Here's how the part is built. I have some questions about the finished solid (model axes, mm). Round coordinates to 2 decimals unless told otherwise and drop trailing zeros. Write each loop counter-clockwise with the first axis right and the second up, starting at its lowest first coordinate (ties: lowest second). Pieces come first, ordered by that corner, then holes. Notation, with made-up numbers: (54.5, 11) -> (75.5, 11) arc R14 cw to (75.5, 23) -> close; hole circle Ø8 at (-25, -5.5). An arc over 180 degrees is marked (long way). Put each result on its own line as item: value. Start each with the question number.
1) If I drill on line 1 along X through (y, z) = (37.5, 9.9); line 2 along Y through (x, z) = (39.5, 12.7); line 3 along Y through (x, z) = (9.5, 11.75), over which ranges is the centre line in solid material (lowest first)? Write a range as [from, to].
2) I want a section at D-D, the plane x = 44. List the corners of the cut face in (y, z) for me, then the cut area to 3 significant figures.
3) I want a section at A-A, the plane x = 19. List the corners of the cut face in (y, z) for me.
4) I want a section at B-B, the plane z = 9.5. Give the number of separate pieces and of enclosed holes in the cut face, then the cut area to 3 significant figures.
5) Will these pins go through, and if not, where does the flat tip stop? P1, Ø0.6, axis at y = 3, z = 9, coming from the +X side; P2, Ø1, axis at y = 38, z = 9, coming from the -X side; P3, Ø3, axis at x = 34, y = 31, coming from the -Z side.
6) I want a section at C-C, the plane x = 106.5. List the corners of the cut face in (y, z) for me.
from build123d import *

# Parameters (mm, degrees)
SKETCH005_W     = 115
SKETCH005_H     = 40
PAD002_DEPTH    = 1
SKETCH006_W     = 5
SKETCH006_H     = 2
PAD003_DEPTH    = 5
SKETCH007_R     = 2
POCKET002_DEPTH = 5
SKETCH008_W     = 26
SKETCH008_H     = 18
POCKET003_DEPTH = 5
SKETCH009_W     = 15
SKETCH009_H     = 3.2
POCKET004_DEPTH = 5
SKETCH010_R     = 1.2
POCKET005_DEPTH = 38.701
FILLET002_R     = 2


with BuildPart() as part:
    # Sketch005 → Pad002 (new body)
    with BuildSketch(Plane.XY):
        with Locations((57.5, 20)):
            Rectangle(SKETCH005_W, SKETCH005_H)
    extrude(amount=PAD002_DEPTH)

    # Sketch006 → Pad003 (join)
    with BuildSketch(Plane(origin=(0, 0, 0), x_dir=(1, 0, 0), z_dir=(0, 0, -1))):
        with Locations((8.5, -2.3)):
            Rectangle(SKETCH006_W, SKETCH006_H)
        with Locations((106.5, -2.3)):
            Rectangle(SKETCH006_W, SKETCH006_H)
        with Locations((106.5, -37.7)):
            Rectangle(SKETCH006_W, SKETCH006_H)
        with Locations((8.5, -37.7)):
            Rectangle(SKETCH006_W, SKETCH006_H)
    extrude(amount=PAD003_DEPTH)

    # Sketch007 (on Face5 of Pad003) → Pocket002 (cut)
    with BuildSketch(Plane.XY.offset(1)):
        with Locations((60.085, 10.835)):
            Circle(SKETCH007_R)
        with Locations((60.085, 26.085)):
            Circle(SKETCH007_R)
        with Locations((74.085, 18.585)):
            Circle(SKETCH007_R)
        with Locations((88.085, 18.585)):
            Circle(SKETCH007_R)
    extrude(amount=-POCKET002_DEPTH, mode=Mode.SUBTRACT)

    # Sketch008 (on Face5 of Pocket002) → Pocket003 (cut)
    with BuildSketch(Plane.XY.offset(1)):
        with Locations((37.75, 19.9)):
            Rectangle(SKETCH008_W, SKETCH008_H)
    extrude(amount=-POCKET003_DEPTH, mode=Mode.SUBTRACT)

    # Sketch009 (on Face5 of Pocket003) → Pocket004 (cut)
    with BuildSketch(Plane.XY.offset(1)):
        with Locations((19.95, 35.87)):
            Rectangle(SKETCH009_W, SKETCH009_H)
    extrude(amount=-POCKET004_DEPTH, mode=Mode.SUBTRACT)

    # Sketch010 (on Face7 of Pocket004) → Pocket005 (cut, through all)
    with BuildSketch(Plane.XZ.offset(-1.3)):
        with Locations((8.5, -2.5)):
            Circle(SKETCH010_R)
        with Locations((106.5, -2.5)):
            Circle(SKETCH010_R)
    extrude(amount=-POCKET005_DEPTH, mode=Mode.SUBTRACT)

    # Fillet002
    fillet002_edges = [part.edges().sort_by_distance(p)[0] for p in [
        (0, 0, 0.5),
        (115, 0, 0.5),
        (115, 40, 0.5),
        (0, 40, 0.5),
    ]]
    fillet(fillet002_edges, radius=FILLET002_R)


with BuildPart() as part_1:
    # Body001 placement: moved
    add(part.part.moved(Location((0, 0, 12))))


solid = part_1.part
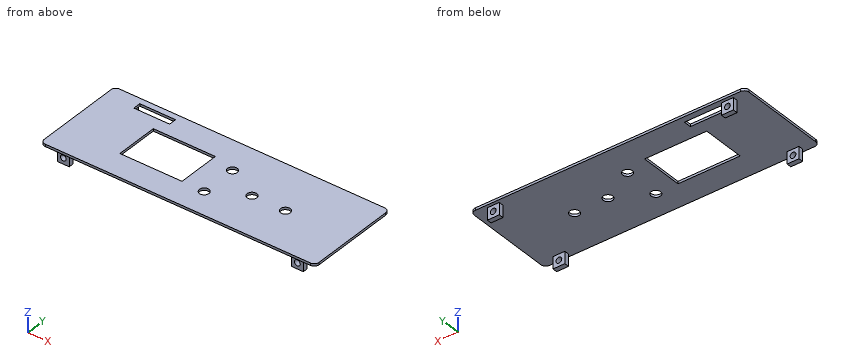
Findings:
1. line 1: x = [6, 7.37], [9.63, 11], [104, 105.37], [107.63, 109]
1. line 2: y = [0, 10.9], [28.9, 40]
1. line 3: y = [1.3, 3.3], [36.7, 38.7]
2. outline: (0, 12) -> (10.9, 12) -> (10.9, 13) -> (0, 13) -> close; (28.9, 12) -> (40, 12) -> (40, 13) -> (28.9, 13) -> close
2. area: 22.0 mm2
3. outline: (0, 12) -> (34.27, 12) -> (34.27, 13) -> (0, 13) -> close; (37.47, 12) -> (40, 12) -> (40, 13) -> (37.47, 13) -> close
4. separate pieces: 8
4. enclosed holes: 0
4. area: 20.8 mm2
5. P1: stops at x = 109
5. P2: stops at x = 6
5. P3: stops at z = 12
6. outline: (0, 12) -> (1.3, 12) -> (1.3, 10.7) -> (3.3, 10.7) -> (3.3, 12) -> (36.7, 12) -> (36.7, 10.7) -> (38.7, 10.7) -> (38.7, 12) -> (40, 12) -> (40, 13) -> (0, 13) -> close; (1.3, 7) -> (3.3, 7) -> (3.3, 8.3) -> (1.3, 8.3) -> close; (36.7, 7) -> (38.7, 7) -> (38.7, 8.3) -> (36.7, 8.3) -> close
